Source: three-view drawing plus pictorial views. Frame: mm from the lowest corner of the part. A direction names the side the tool comes from. Give positions to 0.01 mm unless a question says otherwise; leave off trailing zeros. Loops run counter-clockwise (first coordinate to the right, second up) from the corner with the lowest first, then second, coordinate; pieces in that order, holes last. Notation, with made-up numbers: (52, 74.25) - (79, 74.25) arc R15 ccw to (79, 83.25) - close; hole circle Ø1 at (57.5, 88.25). An arc over 180 degrees is marked (long way). Answer in a Markdown table with one row per item.
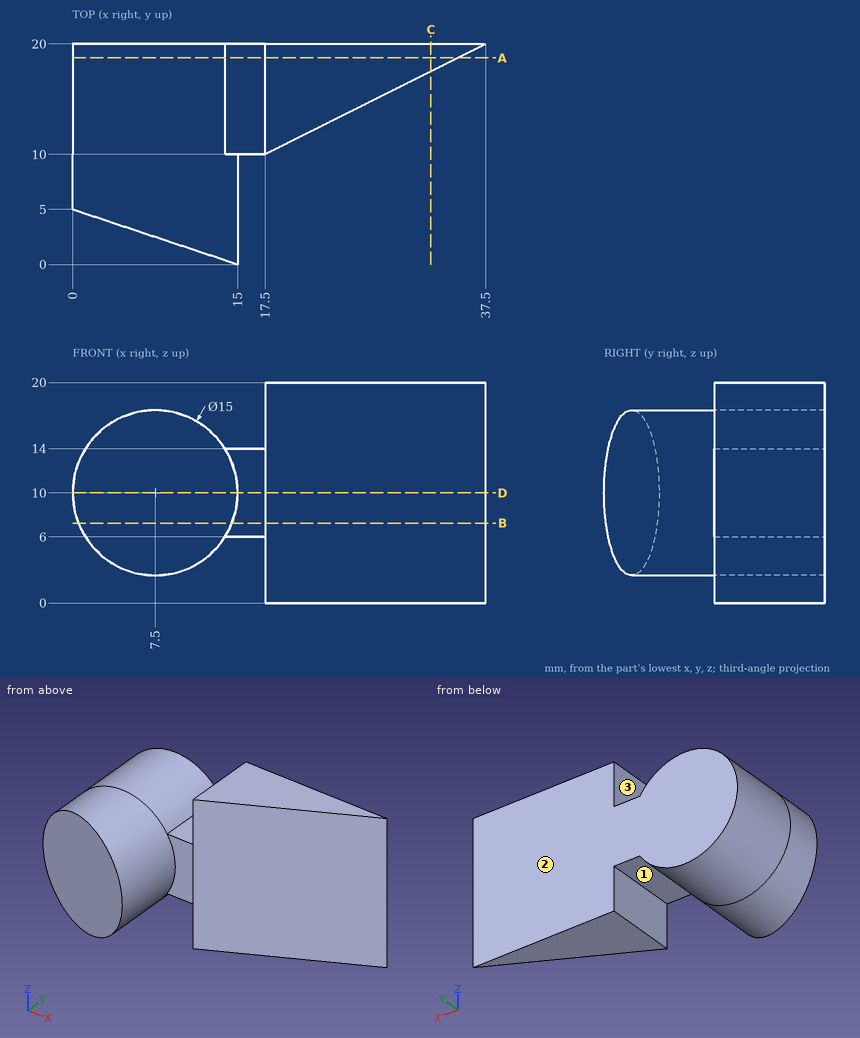
Q1. Cut plane C-C (x = 32.5). Output: boundary loops of the cut face in (y, z), and give its area (3 significant figures).
Check values:
| item | result |
|---|---|
| outline | (17.5, 0) - (20, 0) - (20, 20) - (17.5, 20) - close |
| area | 50.0 mm² |
Q2. First-contact query: pin 1 (12 mm diameter, centred on y = 5, z = 6, fed in from +X); pin 2 (1.1 mm diameter, centred on x = 15, z = 11.5, fed in from -Y); pin 3 (4 mm diameter, centred on y = 2.5, z = 16.5, fed in from -X). Flat tips, straight axial feed; report the tip coordinate or a pass-through.
Check values:
| item | result |
|---|---|
| pin 1 | x = 19.5 |
| pin 2 | y = 0.02 |
| pin 3 | x = 2.36 |
Q3. Cut plane D-D (z = 10). Output: boundary loops of the cut face in (x, y).
Check values:
| item | result |
|---|---|
| outline | (0, 5) - (15, 0) - (15, 10) - (17.5, 10) - (37.5, 20) - (0, 20) - close |
Q4. Material intervals for line 1 along Y through (x, z) = (27.5, 2.75); line 2 along Y through (x, z) = (25.5, 4); line 3 along X through (y, z) = (11.25, 3.75), sorted ascending.
Check values:
| item | result |
|---|---|
| line 1 | 15 to 20 |
| line 2 | 14 to 20 |
| line 3 | 3.35 to 11.65, 17.5 to 20 |
Q5. Cut plane B-B (z = 7.25). Output: boundary loops of the cut face in (x, y).
Check values:
| item | result |
|---|---|
| outline | (0.52, 4.83) - (14.48, 0.17) - (14.48, 10) - (17.5, 10) - (37.5, 20) - (0.52, 20) - close |
Q6. Cut plane A-A (y = 18.75). Output: boundary loops of the cut face in (x, z).
Check values:
| item | result |
|---|---|
| outline | (13.84, 6) - (17.5, 6) - (17.5, 0) - (35, 0) - (35, 20) - (17.5, 20) - (17.5, 14) - (13.84, 14) arc R7.5 ccw (long way) to start |
Q7. Reachability of the marked faces 1, 2 and 3 from +Z, -Z, +X, -X, +Y, -Y: full face, straight path, thin tool, end or side. Return the list, or none.
Check values:
| item | result |
|---|---|
| face 1 | -Z, +Y, -Y |
| face 2 | +Z, -Z, +X, -X, +Y |
| face 3 | +Z, +Y, -Y |
